Verification items for the finished model (mm, model axes). A direction names the side the tool comes from. Give positions to 0.01 mm unless a question says otherwise; leave off trailing zeros. Loops run counter-clockwise (first coordinate to the right, second up) from the corner with the lowest first, then second, coordinate; pieces in that order, holes last. Notation, with made-up numbers: M 56,-23.75 L 62,-23.75 A20 cw 62,-12.75 Z; hole C 84.5,23 d7. An arc over 180 degrees is marked long. Use a Markdown table: item, result.
from build123d import *

# Parameters (mm, degrees)
F1_DEPTH = 3.175
F3_DEPTH = 30.7975
F4_W     = 42.545
F4_H     = 15.24
F5_DEPTH = 3.175
F6_W     = 38.1
F6_H     = 22.86
F7_DEPTH = 48.896
F8_W     = 50.8
F8_H     = 5.08
F9_DEPTH = 6.35
F10_R    = 7.62


with BuildPart() as f1:
    # F0 (on Top) → F1 (new body)
    with BuildSketch(Plane.XY):
        Polygon((-21.1101771393, 107.2532582595), (-32.5401771393, 107.2532582595), (-32.5401771393, -31.9387417405), (13.1798228607, -31.9387417405), (13.1798228607, -19.7467417405), (10.0048228607, -19.7467417405), (10.0048228607, 5.6532582595), (13.1798228607, 5.6532582595), (16.3548228607, 5.6532582595), (16.3548228607, 31.0532582595), (13.1798228607, 31.0532582595), (10.0048228607, 31.0532582595), (10.0048228607, 56.4532582595), (13.1798228607, 56.4532582595), (16.3548228607, 56.4532582595), (16.3548228607, 81.8532582595), (13.1798228607, 81.8532582595), (13.1798228607, 107.2532582595), (10.0048228607, 107.2532582595), (4.2898228607, 107.2532582595), (4.2898228607, 113.6032582595), (-21.1101771393, 113.6032582595), align=None)
    extrude(amount=F1_DEPTH)

    # F2 (on face) → F3 (join)
    with BuildSketch(Plane.XY.offset(3.175)):
        Polygon((13.1798228607, -28.7637417405), (-29.3651771393, -28.7637417405), (-29.3651771393, 107.2532582595), (-32.5401771393, 107.2532582595), (-32.5401771393, -31.9387417405), (13.1798228607, -31.9387417405), align=None)
    extrude(amount=F3_DEPTH)

    # F4 (on face) → F5 (join)
    with BuildSketch(Plane.XY.offset(33.9725)):
        with Locations((-8.0926771393, -21.1437417405)):
            Rectangle(F4_W, F4_H)
    extrude(amount=-F5_DEPTH)

    # F6 (on face) → F7 (cut, through all)
    with BuildSketch(Plane(origin=(-32.5401771393, 0, 0), x_dir=(0, -1, 0), z_dir=(-1, 0, 0))):
        with Locations((-5.5262582595, 22.5425)):
            Rectangle(F6_W, F6_H)
    extrude(amount=-F7_DEPTH, mode=Mode.SUBTRACT)

    # F8 (on face) → F9 (join)
    with BuildSketch(Plane.YZ.offset(-29.3651771393)):
        with Locations((75.3762582595, 15.08125)):
            Rectangle(F8_W, F8_H)
    extrude(amount=F9_DEPTH)

    # F10
    f10_edges = [f1.edges().sort_by_distance(p)[0] for p in [
        (-32.540177, -31.938742, 16.98625),
    ]]
    fillet(f10_edges, radius=F10_R)


solid = f1.part
(1) Cross-section at C-C on z = 9.5. Record the cut outline in (x, y).
Results below:
| item | result |
|---|---|
| outline | M -32.54,-24.32 A7.62 ccw -24.92,-31.94 L 13.18,-31.94 L 13.18,-28.76 L -29.37,-28.76 L -29.37,107.25 L -32.54,107.25 Z |
(2) Draft check along Z on faces 6 (the flat face through (-8, 42, 0)), 7 (the flat face through (-8, -28.764, 17)), 8 (the flat face through (16.355, 18, 2)). Enter one of: +Z half, -Z half, draft (parallel to the pull), parting line (faces both ways), or undercut.
Results below:
| item | result |
|---|---|
| face 6 | -Z half |
| face 7 | undercut |
| face 8 | draft |
(3) Gauge pin test, flat ends, axial feed: P1, Ø8, axis at x = -13, y = 49.5, coming from the +Z side (3 decimals); P2, Ø3, axis at x = -26.5, y = 70, coming from the +Z side; P3, Ø4, axis at y = 82.5, z = 15, coming from the +X side. Record the tip position at first contact, or that the pin passes through.
Results below:
| item | result |
|---|---|
| P1 | z = 3.175 |
| P2 | z = 17.62 |
| P3 | x = -23.02 |
(4) Set-up check for faces 1 (the flat face through (-30, 107.253, 13)), 2 (the flat face through (9, 107.253, 2)), 3 (the flat face through (-31, 24.576, 22)), 4 (the flat face through (10.005, -7, 2)), 5 (the flat face through (10.005, 44, 2)): record each of +Z, -Z, +X, -X, +Y, -Y from which the full face is reachable in a straight line by a thin tool's end or side.
Results below:
| item | result |
|---|---|
| face 1 | +Z, -Z, -X, +Y |
| face 2 | +Z, -Z, +X, +Y |
| face 3 | +Z, +X, -X |
| face 4 | -Z, +X |
| face 5 | +Z, -Z, +X |
(5) Cross-section at B-B on x = -18.5. Record the cut outline in (y, z) (1 decimal), then the cut area to 3 significant figures.
Results below:
| item | result |
|---|---|
| outline | M -31.9,0 L 113.6,0 L 113.6,3.2 L -28.8,3.2 L -28.8,30.8 L -13.5,30.8 L -13.5,34 L -31.9,34 Z |
| area | 608 mm^2 |
(6) Material ranges on line 1 (Z direction, x = -24, y = 55.5) (3 decimals); line 2 (Z direction, x = -2.5, y = -24) (1 decimal); line 3 (Z direction, x = -28.5, y = -3) (3 decimals), recorded low to high.
Results below:
| item | result |
|---|---|
| line 1 | 0 to 3.175, 12.541 to 17.621 |
| line 2 | 0 to 3.2, 30.8 to 34 |
| line 3 | 0 to 3.175 |
(7) Cross-section at A-A on z = 15.5. Record the cut outline in (x, y), then the cut area to 3 significant figures.
Results below:
| item | result |
|---|---|
| outline | M -32.54,-24.32 A7.62 ccw -24.92,-31.94 L 13.18,-31.94 L 13.18,-28.76 L -29.37,-28.76 L -29.37,-13.52 L -32.54,-13.52 Z; M -32.54,24.58 L -29.37,24.58 L -29.37,49.98 L -23.02,49.98 L -23.02,100.78 L -29.37,100.78 L -29.37,107.25 L -32.54,107.25 Z |
| area | 766 mm^2 |
(8) Cross-section at D-D on y = 54. Record the cut outline in (x, z) (1 decimal).
Results below:
| item | result |
|---|---|
| outline | M -32.5,0 L 10,0 L 10,3.2 L -29.4,3.2 L -29.4,12.5 L -23,12.5 L -23,17.6 L -29.4,17.6 L -29.4,34 L -32.5,34 Z |
